```python
from build123d import *

# Parameters (mm, degrees)
SKETCH1_R                                      = 12
SKETCH1_R_2                                    = 1.5
SKETCH1_R_3                                    = 1
BOSS_EXTRUDE1_DEPTH                            = 3
CSK_FOR_M2_FLAT_HEAD_MACHINE_SCREW1_AT_2_COUNT = 2
CSK_FOR_M2_FLAT_HEAD_MACHINE_SCREW1_AT_2_PITCH = 14.142135624
CSK_FOR_M2_FLAT_HEAD_MACHINE_SCREW1_AT_3_COUNT = 2
CSK_FOR_M2_FLAT_HEAD_MACHINE_SCREW1_AT_3_PITCH = 20


with BuildPart() as part:
    # Sketch1 → Boss-Extrude1 (new body)
    with BuildSketch(Plane(origin=(0, 0, 0), x_dir=(1, 0, 0), z_dir=(0, 1, 0))):
        with Locations(Location((0, 0, 0), (0, 0, 270))):
            Circle(SKETCH1_R)
        with Locations(Location((0, 0, 0), (0, 0, 270))):
            Circle(SKETCH1_R_2, mode=Mode.SUBTRACT)
        with Locations(Location((-10, 0, 0), (0, 0, 270))):
            Circle(SKETCH1_R_3, mode=Mode.SUBTRACT)
        with Locations(Location((0, 10, 0), (0, 0, 270))):
            Circle(SKETCH1_R_3, mode=Mode.SUBTRACT)
        with Locations(Location((10, 0, 0), (0, 0, 270))):
            Circle(SKETCH1_R_3, mode=Mode.SUBTRACT)
    extrude(amount=BOSS_EXTRUDE1_DEPTH)

    # Sketch3 → CSK for M2 Flat Head Machine Screw1 (revolve, cut)
    with BuildSketch(Plane(origin=(-10, 3, 0), x_dir=(0, 0, 1), z_dir=(1, 0, 0))):
        Polygon((0, 0), (0, 5.600860619), (1, 5), (1, 1.25), (1.95, 0.3), (1.95, 0), align=None)
    csk_for_m2_flat_head_machine_screw1 = revolve(axis=Axis((-10, 9.35, 0), (0, -1, 0)), mode=Mode.SUBTRACT)

    # CSK for M2 Flat Head Machine Screw1 at 2: CSK for M2 Flat Head Machine Screw1 ×2
    with Locations(*[Vector(0.7071067811865476, 0, -0.7071067811865476) * (i * CSK_FOR_M2_FLAT_HEAD_MACHINE_SCREW1_AT_2_PITCH) for i in range(1, CSK_FOR_M2_FLAT_HEAD_MACHINE_SCREW1_AT_2_COUNT)]):
        add(csk_for_m2_flat_head_machine_screw1, mode=Mode.SUBTRACT)

    # CSK for M2 Flat Head Machine Screw1 at 3: CSK for M2 Flat Head Machine Screw1 ×2
    with Locations(*[(i * CSK_FOR_M2_FLAT_HEAD_MACHINE_SCREW1_AT_3_PITCH, 0, 0) for i in range(1, CSK_FOR_M2_FLAT_HEAD_MACHINE_SCREW1_AT_3_COUNT)]):
        add(csk_for_m2_flat_head_machine_screw1, mode=Mode.SUBTRACT)

    # Sketch5 → CSK for M3 Flat Head Machine Screw1 (revolve, cut)
    with BuildSketch(Plane(origin=(0, 3, 0), x_dir=(0, 0, 1), z_dir=(1, 0, 0))):
        Polygon((0, 0), (0, 5.901290929), (1.5, 5), (1.5, 1.8), (3, 0.3), (3, 0), align=None)
    revolve(axis=Axis((0, 9.35, 0), (0, -1, 0)), mode=Mode.SUBTRACT)


solid = part.part
```
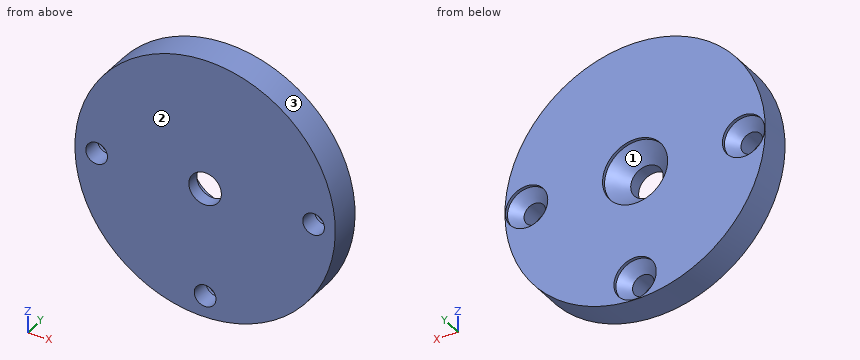
Geometry: final body of the model. Coordinates: model frame, mm. Face numbers are marked on the shaded views. Round coordinates to 2 decimals unless told otherwise and drop trailing zeros. Order: outer loops, then holes, each group sorted by start corner. A loop starts at its lowest first (then second) coordinate and runs counter-clockwise, first axis right, second up. Notation, with made-up numbers: (67.25, 26) - (94.25, 26) arc R18 cw to (94.25, 52) - close; hole circle Ø6 at (32, 31.5). An arc over 180 degrees is marked (long way). Use CSV: the item, a comma, the result in double quotes. Start each with the question number.
Q1. Material intervals for line 1 along X through (y, z) = (1.1, 0); line 2 along Z through (x, y) = (-10.5, 2.15); line 3 along Z through (x, y) = (0.5, 0.45), sorted ascending. Write a range as from..to.
Q2. Section query C-C (z = -10). Return loops of the section in (x, y).
Q3. Mould query, pull axis X, two halves, no side actions, for the marked faces 1, 2 and 3. Classes: +X half, -X half, draft (parallel to the pull), parting line (faces both ways), or undercut.
Q4. Section query B-B (y = 2.15). Return loops of the section in (x, z).
Q5. Section query A-A (z = 0). Return loops of the section in (x, y), and give its area (3 significant figures).
Q6. Section query D-D (x = -10). Return loops of the section in (y, z), and give its area (3 significant figures).
Q7. First-contact query: pin 1 (5.5 mm diameter, centred on x = 0, z = 0, fed in from -Y); pin 2 (1 mm diameter, centred on y = 1, z = -6, fed in from +X); pin 3 (2.5 mm diameter, centred on x = -10, z = 0, fed in from +Y); pin 4 (2.5 mm diameter, centred on x = 0, z = 0, fed in from +Y). Flat tips, straight axial feed; report the tip coordinate or a pass-through.
Result set:
1,line 1,"x = -12..-11, -9..-1.5, 1.5..9, 11..12"
1,line 2,"z = -5.81..-1.31, 1.31..5.81"
1,line 3,"z = -11.99..-10.87, -9.13..-1.41, 1.41..11.99"
2,outline,"(-6.63, 0) - (-1, 0) - (-1, 1.75) - (-1.95, 2.7) - (-1.95, 3) - (-6.63, 3) - close; (1, 0) - (6.63, 0) - (6.63, 3) - (1.95, 3) - (1.95, 2.7) - (1, 1.75) - close"
3,face 1,"undercut"
3,face 2,"draft"
3,face 3,"parting line"
4,outline,"circle Ø24 at (0, 0); hole circle Ø2.8 at (-10, 0); hole circle Ø4.9 at (0, 0); hole circle Ø2.8 at (0, -10); hole circle Ø2.8 at (10, 0)"
5,outline,"(-12, 0) - (-11, 0) - (-11, 1.75) - (-11.95, 2.7) - (-11.95, 3) - (-12, 3) - close; (-9, 0) - (-1.5, 0) - (-1.5, 1.2) - (-3, 2.7) - (-3, 3) - (-8.05, 3) - (-8.05, 2.7) - (-9, 1.75) - close; (1.5, 0) - (9, 0) - (9, 1.75) - (8.05, 2.7) - (8.05, 3) - (3, 3) - (3, 2.7) - (1.5, 1.2) - close; (11, 0) - (12, 0) - (12, 3) - (11.95, 3) - (11.95, 2.7) - (11, 1.75) - close"
5,area,"44.9 mm2"
6,outline,"(0, -6.63) - (3, -6.63) - (3, -1.95) - (2.7, -1.95) - (1.75, -1) - (0, -1) - close; (0, 1) - (1.75, 1) - (2.7, 1.95) - (3, 1.95) - (3, 6.63) - (0, 6.63) - close"
6,area,"32.3 mm2"
7,pin 1,"stops at y = 0"
7,pin 2,"stops at x = 10.67"
7,pin 3,"stops at y = 2"
7,pin 4,"passes through"
